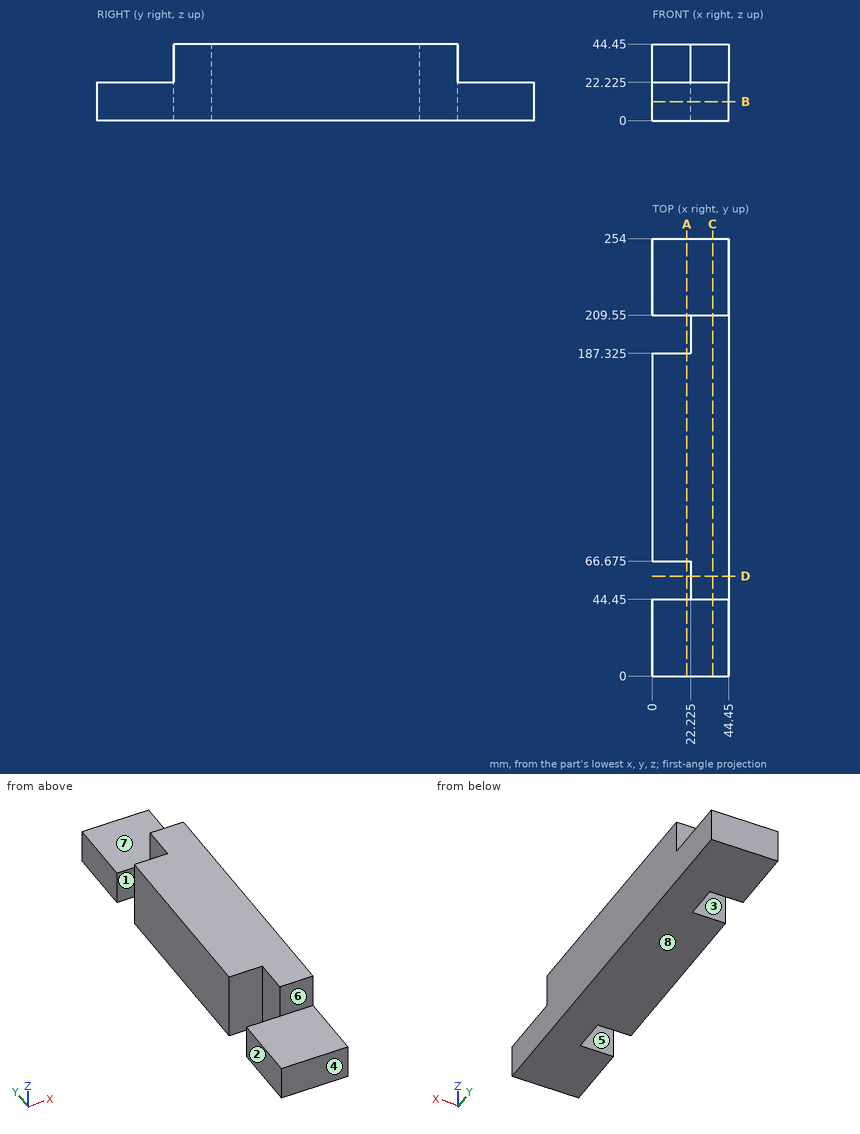
Here's the drawing with two shaded views (mm, measured from the low corner). I have some questions. A direction names the side the tool comes from. Round coordinates to 2 decimals unless told otherwise and drop trailing zeros. Order: outer loops, then holes, each group sorted by start corner. A loop starts at its lowest first (then second) coordinate and runs counter-clockwise, first axis right, second up. Notation, with made-up numbers: (48.5, 87) -> (66.5, 87) arc R22 ccw to (66.5, 115) -> close; hole circle Ø9 at (13.25, 67.5). An arc over 180 degrees is marked (long way). Use a Markdown table: item, result. Add a question column.
(1) Suppose I cut it at C-C, the plane x = 35. Please give me the cut outline in (y, z) (3 decimals), and give its area (3 significant figures).
(2) Suppose I cut it at B-B, the plane z = 11. Please give me the cut outline in (x, y) (3 decimals), and give its area (3 significant figures).
(3) I need wall thicknesses on line 1 along Y through (x, z) = (11.5, 7) (3 decimals); line 2 along Z through (x, y) = (12.5, 226.5) (3 decimals); line 3 along X through (y, z) = (61.5, 9.5) (3 decimals). Which ranges of each line are inside material? Lowest first, please.
(4) If we mould it in two halves opening along Y, with no side actions, what happens to the marked faces 1, 2, 3 and 4? For each: released by +Y, released by -Y, zero draft, split by the parting line, or undercut.
(5) Suppose I cut it at D-D, the plane y = 58. Please give me the cut outline in (x, z) (3 decimals), and give its area (3 significant figures).
(6) For pin 1 Ø24.5 at (x, z) = (30.5, 35) entering from +Y; pin 2 Ø3 at (y, z) = (65, 33.5) entering from -X (3 decimals); pin 3 Ø18 at (x, z) = (31.5, 36) entering from -Y, each with a flat end and sliding along its axis, tell me the tip position at first contact or that it passes through.
(7) Suppose I cut it at A-A, the plane x = 20. Please give me the cut outline in (y, z) (3 decimals), and give its area (3 significant figures).
(8) For the marked faces 5, 6, 7 and 8, which set-ups out of +Z, -Z, +X, -X, +Y, -Y let a thin tool reach every point of the face, with its end or its side?
Verdict:
| question | item | result |
|---|---|---|
| 1 | outline | (0, 0) -> (254, 0) -> (254, 22.225) -> (209.55, 22.225) -> (209.55, 44.45) -> (44.45, 44.45) -> (44.45, 22.225) -> (0, 22.225) -> close |
| 1 | area | 9,310 mm2 |
| 2 | outline | (0, 0) -> (44.45, 0) -> (44.45, 254) -> (0, 254) -> (0, 209.55) -> (22.225, 209.55) -> (22.225, 187.325) -> (0, 187.325) -> (0, 66.675) -> (22.225, 66.675) -> (22.225, 44.45) -> (0, 44.45) -> close |
| 2 | area | 10,300 mm2 |
| 3 | line 1 | 0 to 44.45, 66.675 to 187.325, 209.55 to 254 |
| 3 | line 2 | 0 to 22.225 |
| 3 | line 3 | 22.225 to 44.45 |
| 4 | face 1 | undercut |
| 4 | face 2 | zero draft |
| 4 | face 3 | undercut |
| 4 | face 4 | released by -Y |
| 5 | outline | (22.225, 0) -> (44.45, 0) -> (44.45, 44.45) -> (22.225, 44.45) -> close |
| 5 | area | 988 mm2 |
| 6 | pin 1 | y = 209.55 |
| 6 | pin 2 | x = 22.225 |
| 6 | pin 3 | y = 44.45 |
| 7 | outline | (0, 0) -> (44.45, 0) -> (44.45, 22.225) -> (0, 22.225) -> close; (66.675, 0) -> (187.325, 0) -> (187.325, 44.45) -> (66.675, 44.45) -> close; (209.55, 0) -> (254, 0) -> (254, 22.225) -> (209.55, 22.225) -> close |
| 7 | area | 7,340 mm2 |
| 8 | face 5 | +Z, -Z, -X |
| 8 | face 6 | +Z, +X, -X, -Y |
| 8 | face 7 | +Z, +X, -X, +Y |
| 8 | face 8 | -Z, +X, -X, +Y, -Y |
